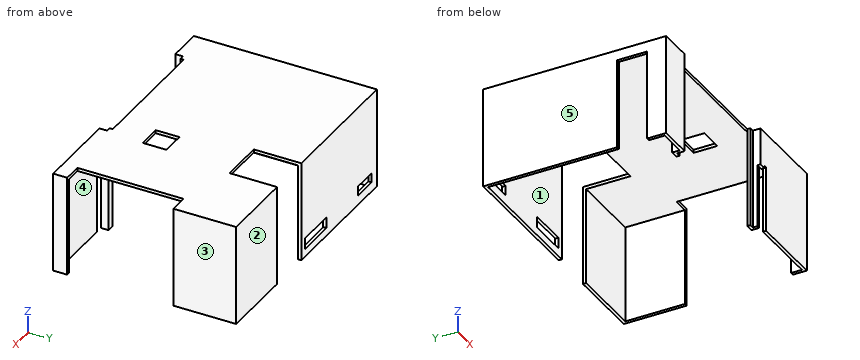
Autodesk Fusion 360 part; units mm, degrees
ref_plane "Arbeitsebene1" through (-71.75, -25.15, 142.25) normal (0, 0, 1) x (0, -1, 0)
sketch "Skizze1" plane through (0, 0, 142.25) normal (0, 0, 1) x (1, 0, 0)
  line L0 (-35.7, -26.35) -> (-35.7, -31.2)
  line L1 (-35.7, -26.35) -> (-40.5, -26.35)
  line L2 (-40.5, -26.35) -> (-40.5, -28.35)
  line L3 (-35.5, -1) -> (-35.5, -31)
  line L4 (-33.5, -26.15) -> (-40.5, -26.15)
  line L5 (-40.5, -28.35) -> (-37.7, -28.35)
  line L6 (-37.7, -28.35) -> (-37.7, -33.2)
  line L7 (-37.7, -33.2) -> (15.7, -33.2)
  line L8 (-35.7, -31.2) -> (13.7, -31.2)
  line L9 (15.7, -33.2) -> (15.7, 82.2)
  line L10 (-127.3, -26.35) -> (-127.3, -31.2)
  line L11 (-127.3, -26.35) -> (-122.5, -26.35)
  line L12 (-103, -26.15) -> (-129.5, -26.15)
  line L13 (-127.5, -1) -> (-127.5, -31)
  line L14 (-122.5, -26.35) -> (-122.5, -28.35)
  line L15 (-122.5, -28.35) -> (-125.3, -28.35)
  line L16 (-125.3, -28.35) -> (-125.3, -33.2)
  line L17 (-125.3, -33.2) -> (-146.7, -33.2)
  line L18 (-127.3, -31.2) -> (-144.7, -31.2)
  line L19 (-144.7, -31.2) -> (-144.7, 80.2)
  line L20 (-146.7, -33.2) -> (-146.7, 82.2)
  line L21 (15.7, 82.2) -> (-146.7, 82.2)
  line L22 (-144.7, 80.2) -> (13.7, 80.2)
  line L23 (13.7, -31.2) -> (13.7, 80.2)
  line L24 (-122.5, -26.35) -> (-40.5, -26.35)
  dimension "d51" = 0.2
  dimension "d52" = 0.2
  dimension "d53" = 4.8
  dimension "d54" = 2
  dimension "d55" = 4.85
  dimension "d56" = 2.8
  dimension "d57" = 4.85
  dimension "d58" = 53.4
  dimension "d59" = 49.4
  dimension "d60" = 115.4
  dimension "d61" = 0.2
  dimension "d62" = 0.2
  dimension "d63" = 4.8
  dimension "d64" = 4.85
  dimension "d65" = 2
  dimension "d66" = 2.8
  dimension "d67" = 4.85
  dimension "d68" = 21.4
  dimension "d69" = 17.4
  dimension "d70" = 111.4
  dimension "d71" = 115.4
  dimension "d72" = 158.4
  dimension "d73" = 162.4
  dimension "d74" = 111.4
extrude "Extrusion1" add sketch "Skizze1" along normal blind 2
extrude "Extrusion2" add sketch "Skizze1" against normal blind 61.5 contours L0 L1 L2 L5 L6 L7 L8 L9 L10 L11 L14 L15 L16 L17 L18 L19 L20 L21 L22 L23
box "Grundkörper Quader5" cut length 67 width 11.65 height -63.5 placed x (0, 1, 0) y (1, 0, 0) z (0, 0, -1) at (4.05, -24.3544, 80.75)
box "Grundkörper Quader1" cut length 40 width 2 height -41.5 placed x (0, -1, 0) y (-1, 0, 0) z (0, 0, -1) at (-31.3, 6.7996, 80.75)
box "Grundkörper Quader2" cut length 2 width 4.4 height -40 placed x (0, 1, 0) y (1, 0, 0) z (0, 0, -1) at (-37.7, -33.2, 80.75)
sketch "Skizze10" plane through (0, 82.2, 0) normal (0, 1, 0) x (-1, 0, 0)
  line L0 (146.7, 80.75) -> (146.7, 144.25)
  line L1 (146.7, 144.25) -> (-15.7, 144.25)
  line L2 (-15.7, 144.25) -> (-15.7, 80.75)
  line L3 (-15.7, 80.75) -> (146.7, 80.75)
  line L4 (146.7, 80.75) -> (124.7, 80.75) construction
  line L5 (124.7, 80.75) -> (124.7, 92.75) construction
  line L6 (124.7, 92.75) -> (146.7, 92.75) construction
  line L7 (146.7, 92.75) -> (146.7, 80.75) construction
  line L8 (146.7, 80.75) -> (140.7, 80.75) construction
  line L9 (140.7, 80.75) -> (140.7, 86.75) construction
  line L10 (140.7, 86.75) -> (146.7, 86.75) construction
  line L11 (146.7, 86.75) -> (146.7, 80.75) construction
  line L12 (140.7, 86.75) -> (124.7, 86.75)
  line L13 (124.7, 86.75) -> (124.7, 92.75)
  line L14 (124.7, 92.75) -> (140.7, 92.75)
  line L15 (140.7, 92.75) -> (140.7, 86.75)
  line L16 (58.5044, 80.75) -> (88.5044, 80.75) construction
  line L17 (88.5044, 80.75) -> (88.5044, 92.75) construction
  line L18 (88.5044, 92.75) -> (58.5044, 92.75) construction
  line L19 (58.5044, 92.75) -> (58.5044, 80.75) construction
  line L20 (58.5044, 80.75) -> (63.5044, 80.75) construction
  line L21 (63.5044, 80.75) -> (63.5044, 85.75) construction
  line L22 (63.5044, 85.75) -> (58.5044, 85.75) construction
  line L23 (58.5044, 85.75) -> (58.5044, 80.75) construction
  line L24 (63.5044, 85.75) -> (88.5044, 85.75)
  line L25 (88.5044, 85.75) -> (88.5044, 92.75)
  line L26 (88.5044, 92.75) -> (63.5044, 92.75)
  line L27 (63.5044, 92.75) -> (63.5044, 85.75)
  dimension "d87" = 22
  dimension "d88" = 12
  dimension "d89" = 6
  dimension "d90" = 6
  dimension "d93" = 30
  dimension "d94" = 12
  dimension "d95" = 5
  dimension "d96" = 5
extrude "Extrusion3" cut sketch "Skizze10" against normal blind 2 contours L12 L13 L14 L15 | L24 L25 L26 L27
box "Grundkörper Quader3" cut length 30 width 28 height -63.5 placed x (0, 1, 0) y (1, 0, 0) z (0, 0, -1) at (-59.529, 52.2, 80.75)
box "Grundkörper Quader4" cut length 15 width 15 height -2 placed x (0, -1, 0) y (1, 0, 0) z (0, 0, 1) at (-51, 10, 144.25)
sketch "Skizze14" plane through (-146.7, 0, 0) normal (-1, 0, 0) x (0, -1, 0)
  line L0 (33.2, 80.75) -> (33.2, 144.25)
  line L1 (33.2, 144.25) -> (-82.2, 144.25)
  line L2 (-82.2, 144.25) -> (-82.2, 80.75)
  line L3 (-82.2, 80.75) -> (33.2, 80.75)
  line L4 (33.2, 80.75) -> (21.2, 80.75) construction
  line L5 (33.2, 80.75) -> (2.2, 80.75) construction
  line L6 (2.2, 80.75) -> (2.2, 137.75) construction
  line L7 (2.2, 137.75) -> (33.2, 137.75) construction
  line L8 (33.2, 137.75) -> (33.2, 80.75) construction
  line L9 (21.2, 80.75) -> (2.2, 80.75)
  line L10 (2.2, 80.75) -> (2.2, 137.75)
  line L11 (2.2, 137.75) -> (21.2, 137.75)
  line L12 (21.2, 137.75) -> (21.2, 80.75)
  dimension "d112" = 12
  dimension "d114" = 31
  dimension "d115" = 57
extrude "Extrusion4" cut sketch "Skizze14" against normal blind 2 contours L3 L9 L10 L11 L12
Can you work these out from the model? Positions are in its coordinate system, mm. Face numbers are marked on the shaded views. A direction names the side the tool comes from. Coordinates: 2 decimals unless noted, no trailing zeros. Loops run counter-clockwise (first coordinate to the right, second up) from the corner with the lowest first, then second, coordinate; pieces in that order, holes last. Notation, with made-up numbers: M 42,33 L 91,33 A28 ccw 91,69 Z; hole C 81.5,2.5 d7. An arc over 180 degrees is marked long. Answer as CSV lines item,"result". Start each with the question number.
1. Suppose I cut it at C-C, the plane z = 113.5. Count the separate pieces of the cut face and the enclosed holes in it, plus the area to 3 significant figures.
2. If I drill on probe 1 along X at (y, z) = (62.5, 138); probe 2 along Y at (x, z) = (-137.5, 138.5); probe 3 along Z at (x, y) = (3.5, 41.5), over which ranges is the centre line in solid material (lowest first)? Write a range as [from, to].
3. For the marked faces 4 and 5, which set-ups out of +Z, -Z, +X, -X, +Y, -Y let a thin tool reach every point of the face, with its end or its side?
4. For pin 1 Ø1.6 at (x, z) = (-36.5, 108.5) entering from -Y; pin 2 Ø12 at (y, z) = (5, 115.5) entering from +X; pin 3 Ø1 at (x, z) = (-46, 143.5) entering from +Y, each with a flat end and sliding along its axis, tell me the tip position at first contact or that it passes through.
5. Suppose I cut it at B-B, the plane y = 54. List the corners of the cut face in (x, z) for me.
6. Suppose I cut it at D-D, the plane x = 1.5. List the corners of the cut face in (y, z) for me, plus the area to 3 significant figures.
7. Suppose I cut it at A-A, the plane x = -45. List the corners of the cut face in (y, z) for me.
8. Thinking about a two-plate mould opening in X: for the marked faces 1, 2 and 3, which applies, +X half, -X half, draft (parallel to the pull), parting line (faces both ways), or undercut?
Output:
1,separate pieces,"5"
1,enclosed holes,"0"
1,area,"710 mm^2"
2,probe 1,"x = [-146.7, -144.7], [13.7, 15.7]"
2,probe 2,"y = [-33.2, -31.2], [80.2, 82.2]"
2,probe 3,"z = [142.25, 144.25]"
3,face 4,"-Z"
3,face 5,"+Z, -Z, -X, +Y, -Y"
4,pin 1,"stops at y = -31.2"
4,pin 2,"stops at x = -144.7"
4,pin 3,"stops at y = 52.2"
5,outline,"M -146.7,80.75 L -144.7,80.75 L -144.7,142.25 L -59.53,142.25 L -59.53,144.25 L -146.7,144.25 Z; M -31.53,142.25 L 13.7,142.25 L 13.7,80.75 L 15.7,80.75 L 15.7,144.25 L -31.53,144.25 Z"
6,outline,"M -33.2,80.75 L -31.2,80.75 L -31.2,142.25 L 80.2,142.25 L 80.2,80.75 L 82.2,80.75 L 82.2,144.25 L -33.2,144.25 Z"
6,area,"477 mm^2"
7,outline,"M -26.35,142.25 L -5,142.25 L -5,144.25 L -26.35,144.25 Z; M 10,142.25 L 52.2,142.25 L 52.2,144.25 L 10,144.25 Z"
8,face 1,"undercut"
8,face 2,"draft"
8,face 3,"+X half"
